from build123d import *

# Parameters (mm, degrees)
SKETCH3_R           = 2.25
BOSS_EXTRUDE1_DEPTH = 15
CUT_EXTRUDE2_DEPTH  = 5.25
CUT_EXTRUDE3_DEPTH  = 5.25
SKETCH9_W           = 4.986330716
SKETCH9_H           = 10
CUT_EXTRUDE4_DEPTH  = 20


with BuildPart() as part:
    # Sketch3 → Boss-Extrude1 (new body)
    with BuildSketch(Plane.XY):
        with BuildLine():
            Line((-83.240837696, 45.680087808), (-86.318243263, 88.806933971))
            ThreePointArc((-86.318243263, 88.806933971), (-38.505178909, 149.199689366), (30.717635907, 115.412473794))
            ThreePointArc((30.717635907, 115.412473794), (32.594544712, 111.314313071), (34.392132503, 107.180744866))
            ThreePointArc((34.392132503, 107.180744866), (38.03694462, 105.671014255), (41.681756737, 107.180744866))
            Line((41.681756737, 107.180744866), (41.681756737, 115.412473794))
            ThreePointArc((41.681756737, 115.412473794), (8.630903534, 145.599759454), (-35.251645513, 154.428859194))
            ThreePointArc((-35.251645513, 154.428859194), (-74.611345825, 131.314701457), (-91.240837696, 88.806933971))
            Line((-91.240837696, 88.806933971), (-91.240837696, 47.654450262))
            Line((-91.240837696, 47.654450262), (-91.240837696, 39.931378559))
            Line((-91.240837696, 39.931378559), (-83.240837696, 39.931378559))
            Line((-83.240837696, 39.931378559), (-83.240837696, 45.680087808))
        make_face()
        with Locations((-87.125618482, 43.130480477)):
            Circle(SKETCH3_R, mode=Mode.SUBTRACT)
        with Locations((37.681756737, 110.446980465)):
            Circle(SKETCH3_R, mode=Mode.SUBTRACT)
    extrude(amount=-BOSS_EXTRUDE1_DEPTH)

    # Sketch5 → Cut-Extrude2 (cut)
    with BuildSketch(Plane.XY):
        Polygon((-91.240837696, 47.634728669), (-83.240837696, 45.336049347), (-83.240837696, 39.931378559), (-91.240837696, 39.931378559), align=None)
    extrude(amount=-CUT_EXTRUDE2_DEPTH, mode=Mode.SUBTRACT)

    # Sketch8 → Cut-Extrude3 (cut)
    with BuildSketch(Plane(origin=(0, 0, -15), x_dir=(-1, 0, 0), z_dir=(0, 0, -1))):
        Polygon((91.240837696, 47.718881947), (83.240837696, 45.410478658), (83.240837696, 39.931378559), (91.240837696, 39.931378559), align=None)
    extrude(amount=-CUT_EXTRUDE3_DEPTH, mode=Mode.SUBTRACT)

    # Sketch9 → Cut-Extrude4 (cut)
    with BuildSketch(Plane(origin=(41.681756737, 0, 0), x_dir=(0, 0, -1), z_dir=(1, 0, 0))):
        with Locations((7.506834642, 110.671014255)):
            Rectangle(SKETCH9_W, SKETCH9_H)
    extrude(amount=-CUT_EXTRUDE4_DEPTH, mode=Mode.SUBTRACT)


solid = part.part
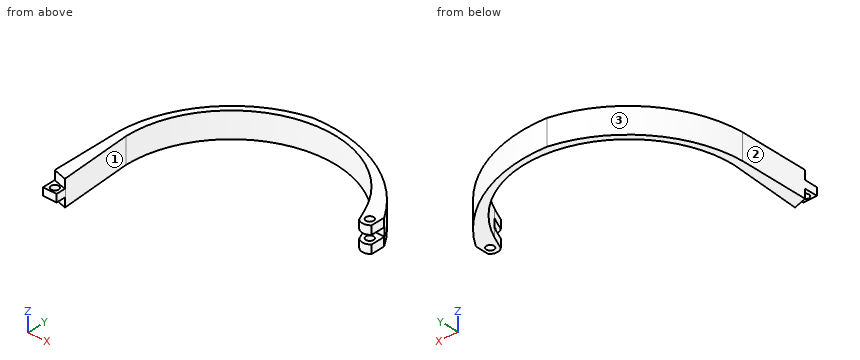
Input: part model. Units: mm. Frame: model coordinates. Face numbers are marked on the shaded views. Coordinates: 2 decimals unless noted, no trailing zeros. Loops run counter-clockwise (first coordinate to the right, second up) from the corner with the lowest first, then second, coordinate; pieces in that order, holes last. Notation, with made-up numbers: (44.5, 10) -> (48.5, 10) arc R23 cw to (48.5, 27) -> close; hole circle Ø2 at (-7, 54.25). An arc over 180 degrees is marked (long way). Write each question's results on one line, items separated by ' | '. Start each with the question number.
Q1. Section A-A, the plane y = 144. Return the cut outline in (x, z).
Q2. Ray query, line 1 (X direction, y = 134.5, z = -8.75); line 2 (X direction, y = 135, z = -5.5); line 3 (Y direction, x = -3.5, z = -13.5). Return the intervals inside material, ascending. Write a range as from..to.
Q3. Section B-B, the plane z = -2.25. Return the cut outline in (x, y), plus the area to 3 significant figures.
Q4. Section D-D, the plane y = 92.5. Return the cut outline in (x, z).
Q5. Section C-C, the plane x = 7. Return the cut outline in (y, z), plus the area to 3 significant figures.
Q6. Pull-direction query (Y, two-part tool) for the marked faces 1, 2 and 3; classes: released by +Y, released by -Y, zero draft, split by the parting line, or undercut.
Q7. Pin query (flat end, axial travel): pin 1 (4 mm diameter, centred on x = -87.5, y = 43.5, fed in from -Z); pin 2 (3 mm diameter, centred on x = -41, z = -2.5, fed in from -Y); pin 3 (4 mm diameter, centred on x = 38, z = -8.5, fed in from -Y). Return the tip coordinate at first contact, or that it passes through.
Found:
1) outline: (-60.36, -15) -> (-52.84, -15) -> (-52.84, 0) -> (-60.36, 0) -> close; (3.07, -15) -> (11.63, -15) -> (11.63, 0) -> (3.07, 0) -> close
2) line 1: -71.72..-66.49, 16.71..25.24 | line 2: -71.23..-65.94, 16.16..24.65 | line 3: 146.89..150.6
3) outline: (-91.24, 47.63) -> (-83.24, 45.34) -> (-83.24, 45.68) -> (-86.32, 88.81) arc R61.43 cw to (30.72, 115.41) arc R233.9 cw to (34.39, 107.18) arc R5.15 ccw to (41.68, 107.18) -> (41.68, 115.41) arc R83.67 ccw to (-35.25, 154.43) arc R69.73 ccw to (-91.24, 88.81) -> close; hole circle Ø4.5 at (37.68, 110.45) | area: 1,130 mm2
4) outline: (-91, -15) -> (-86.24, -15) -> (-86.24, 0) -> (-91, 0) -> close
5) outline: (141.8, -15) -> (146.4, -15) -> (146.4, 0) -> (141.8, 0) -> close | area: 69.0 mm2
6) face 1: undercut | face 2: zero draft | face 3: released by +Y
7) pin 1: z = -9.75 | pin 2: y = 148.15 | pin 3: y = 105.67
